Read the model definition and answer for the solid it produces. Units are mm, in the model's axes. Face numbers are marked on the shaded views. A direction names the side the tool comes from. Give positions to 0.01 mm unless a question says otherwise; leave off trailing zeros. Loops run counter-clockwise (first coordinate to the right, second up) from the corner with the lowest first, then second, coordinate; pieces in that order, holes last. Notation, with made-up numbers: (32.25, -5.75) - (85.25, -5.75) arc R22 cw to (85.25, 0.25) - close; hole circle Ø7 at (-10.5, -10). An arc over 180 degrees is marked (long way). Write item = value, one per line.
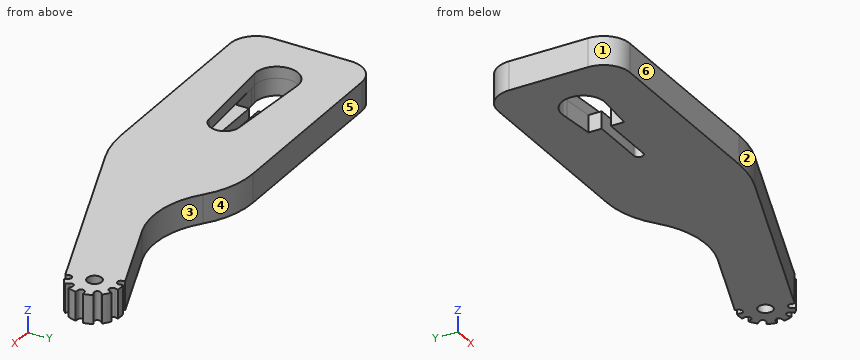
```python
from build123d import *
from build123d.topology import SkipClean

# Parameters (mm, degrees)
CROQUIS1_R              = 1.717841821
CROQUIS1_R_2            = 1.259750669
CROQUIS1_W              = 27.485469141
CROQUIS1_H              = 14.887962451
SALIENTE_EXTRUIR1_DEPTH = 5
SALIENTE_EXTRUIR2_START = -5
SALIENTE_EXTRUIR2_DEPTH = 5
CORTAR_EXTRUIR1_DEPTH   = 5
CORTAR_EXTRUIR2_DEPTH   = 2
CUT_EXTRUDE2_DEPTH      = 83.704538261
CUT_EXTRUDE5_DEPTH      = 83.704538261


with BuildPart() as part:
    # Croquis1 → Saliente-Extruir1 (new body)
    with BuildSketch(Plane(origin=(0, 0, -2.5), x_dir=(-1, 0, 0), z_dir=(0, 0, -1))):
        with BuildLine():
            Line((2.183126414, 10.199004786), (2.457799007, 10.747834714))
            ThreePointArc((2.457799007, 10.747834714), (3.150356623, 11.03498533), (3.533498829, 10.390552574))
            Line((3.533498829, 10.390552574), (3.410556906, 9.704532228))
            Line((3.410556906, 9.704532228), (36.957948904, -3.17310503))
            ThreePointArc((36.957948904, -3.17310503), (40.309989238, -4.118478177), (43.778179918, -4.437160132))
            Line((43.778179918, -4.437160132), (75.884737747, -4.437160132))
            ThreePointArc((75.884737747, -4.437160132), (79.123931349, -3.095442211), (80.46564927, 0.143751392))
            Line((80.46564927, 0.143751392), (80.46564927, 13.886485962))
            ThreePointArc((80.46564927, 13.886485962), (79.123931349, 17.125679564), (75.884737747, 18.467397485))
            Line((75.884737747, 18.467397485), (43.778179918, 18.467397485))
            ThreePointArc((43.778179918, 18.467397485), (38.923372817, 17.631925595), (34.62713443, 15.221634951))
            ThreePointArc((34.62713443, 15.221634951), (27.84817952, 12.197288027), (20.46564927, 12.971336544))
            Line((20.46564927, 12.971336544), (6.293279019, 18.411599775))
            Line((6.293279019, 18.411599775), (6.008822105, 17.843219559))
            ThreePointArc((6.008822105, 17.843219559), (5.316264489, 17.556068943), (4.933122282, 18.200501699))
            Line((4.933122282, 18.200501699), (5.041383533, 18.804603367))
            ThreePointArc((5.041383533, 18.804603367), (4.263160644, 18.876341405), (3.484068945, 18.814751339))
            Line((3.484068945, 18.814751339), (3.584448287, 18.209290101))
            ThreePointArc((3.584448287, 18.209290101), (3.192940304, 17.56990522), (2.504183677, 17.866056933))
            Line((2.504183677, 17.866056933), (2.236686818, 18.418419815))
            ThreePointArc((2.236686818, 18.418419815), (1.564924714, 18.019029169), (0.970828021, 17.511263148))
            Line((0.970828021, 17.511263148), (1.407917802, 17.080436215))
            ThreePointArc((1.407917802, 17.080436215), (1.467002194, 16.333040361), (0.735712768, 16.167791142))
            Line((0.735712768, 16.167791142), (0.194632507, 16.457431391))
            ThreePointArc((0.194632507, 16.457431391), (-0.114078519, 15.739465714), (-0.296255461, 14.9794731))
            Line((-0.296255461, 14.9794731), (0.310591317, 14.887841716))
            ThreePointArc((0.310591317, 14.887841716), (0.797699855, 14.317914702), (0.303205335, 13.754384137))
            Line((0.303205335, 13.754384137), (-0.304784058, 13.670669023))
            ThreePointArc((-0.304784058, 13.670669023), (-0.132526888, 12.9083668), (0.16680132, 12.18643894))
            Line((0.16680132, 12.18643894), (0.711610253, 12.469003179))
            ThreePointArc((0.711610253, 12.469003179), (1.440684032, 12.294237755), (1.371864517, 11.547675365))
            Line((1.371864517, 11.547675365), (0.929197275, 11.122581216))
            ThreePointArc((0.929197275, 11.122581216), (1.516626257, 10.607115987), (2.183126414, 10.199004786))
        make_face()
        with Locations(Location((46.05155145, 7.015118677, 0), (0, 0, 180))):
            Circle(CROQUIS1_R, mode=Mode.SUBTRACT)
        with Locations(Location((77.659840962, 7.015118677, 0), (0, 0, 180))):
            Circle(CROQUIS1_R, mode=Mode.SUBTRACT)
        with Locations(Location((4.233310556, 14.295527136, 0), (0, 0, 180))):
            Circle(CROQUIS1_R_2, mode=Mode.SUBTRACT)
        with Locations((61.855696206, 7.015118677)):
            Rectangle(CROQUIS1_W, CROQUIS1_H, mode=Mode.SUBTRACT)
    extrude(amount=-SALIENTE_EXTRUIR1_DEPTH)

    # Croquis2 → Saliente-Extruir2 (add)
    with BuildSketch(Plane.XY.offset(2.5).offset(SALIENTE_EXTRUIR2_START)):
        with BuildLine():
            Line((-43.778179918, -4.437160132), (-75.884737747, -4.437160132))
            ThreePointArc((-75.884737747, -4.437160132), (-79.123931349, -3.095442211), (-80.46564927, 0.143751392))
            Line((-80.46564927, 0.143751392), (-80.46564927, 13.886485962))
            ThreePointArc((-80.46564927, 13.886485962), (-79.123931349, 17.125679564), (-75.884737747, 18.467397485))
            Line((-75.884737747, 18.467397485), (-43.778179918, 18.467397485))
            Line((-43.778179918, 18.467397485), (-43.778179918, -4.437160132))
        make_face()
    extrude(amount=SALIENTE_EXTRUIR2_DEPTH)

    # Croquis3 → Cortar-Extruir1 (cut)
    with BuildSketch(Plane.XY.offset(2.5)):
        with BuildLine():
            Line((-68.86564927, 10.615118677), (-63.46564927, 10.110118677))
            Line((-63.46564927, 10.110118677), (-63.46564927, 3.920118677))
            Line((-63.46564927, 3.920118677), (-68.86564927, 3.415118677))
            ThreePointArc((-68.86564927, 3.415118677), (-72.46564927, 7.015118677), (-68.86564927, 10.615118677))
        make_face()
    extrude(amount=-CORTAR_EXTRUIR1_DEPTH, mode=Mode.SUBTRACT)

    # Croquis4 → Cortar-Extruir2 (cut)
    with BuildSketch(Plane.XY.offset(2.5)):
        with BuildLine():
            Line((-54.77859891, 9.608381518), (-69.913267682, 10.700035319))
            ThreePointArc((-69.913267682, 10.700035319), (-73.947018097, 7.015118677), (-69.913267682, 3.330202034))
            Line((-69.913267682, 3.330202034), (-54.77859891, 4.421855836))
            ThreePointArc((-54.77859891, 4.421855836), (-52.36564927, 7.015118677), (-54.77859891, 9.608381518))
        make_face()
    extrude(amount=-CORTAR_EXTRUIR2_DEPTH, mode=Mode.SUBTRACT)

    # Sketch2 → Cut-Extrude2 (cut, through all)
    with SkipClean():  # the faces are left unmerged after this step: merging them gives an invalid solid
        with BuildSketch(Plane.XY.offset(0.5)):
            with BuildLine():
                Line((-69.913267682, 10.700035319), (-68.86564927, 10.615118677))
                ThreePointArc((-68.86564927, 10.615118677), (-72.46564927, 7.015118677), (-68.86564927, 3.415118677))
                Line((-68.86564927, 3.415118677), (-69.913267682, 3.330202034))
                ThreePointArc((-69.913267682, 3.330202034), (-73.947018097, 7.015118677), (-69.913267682, 10.700035319))
            make_face()
        extrude(amount=-CUT_EXTRUDE2_DEPTH, mode=Mode.SUBTRACT)

    # Sketch5 → Cut-Extrude5 (cut, through all)
    with SkipClean():  # the faces are left unmerged after this step: merging them gives an invalid solid
        with BuildSketch(Plane.XY.offset(0.5)):
            with BuildLine():
                Line((-63.46564927, 7.815118677), (-53.96564927, 7.815118677))
                ThreePointArc((-53.96564927, 7.815118677), (-53.16564927, 7.015118677), (-53.96564927, 6.215118677))
                Line((-53.96564927, 6.215118677), (-63.46564927, 6.215118677))
                Line((-63.46564927, 6.215118677), (-63.46564927, 7.815118677))
            make_face()
        extrude(amount=-CUT_EXTRUDE5_DEPTH, mode=Mode.SUBTRACT)


solid = part.part
```
1) The mould has two halves that part along X. Classify the marked faces 1, 2, 3 and 4: pulls with the +X half, pulls with the -X half, needs draft (parallel to the pull), parting line crosses it, or undercut.
Output:
face_1 = pulls with the -X half
face_2 = pulls with the +X half
face_3 = undercut
face_4 = undercut
2) Find the intervals of material crossed by probe 1 along Y at (x, z) = (-74.5, 0.65); probe 2 along X at (y, z) = (11, 1.1); probe 3 along X at (y, z) = (10, -1.35), in increasing order.
Output:
probe_1 = -4.44 to 18.47
probe_2 = -80.47 to -3.23, -2.71 to -1.05
probe_3 = -80.47 to -72.43, -63.47 to -3.46
3) A tool of negligible diameter and unlimited length cuts with its end or side. For the marked faces 5 and 6, from which of +Z, -Z, +X, -X, +Y, -Y can it reach the whole face along a straight path? Write none if from no direction.
Output:
face_5 = +Z, -Z, -X, +Y
face_6 = +Z, -Z, +X, -X, -Y
4) A cutting plane is placed at B-B on z = -0.45. Give the number of separate pieces and of enclosed holes in the cut face, then the cut area to 3 significant figures.
Output:
separate_pieces = 1
enclosed_holes = 2
area = 1,300 mm²
5) Each of these flat-tipped pins is pushed along its axis until it touches: P1, Ø8.5, axis at x = -70.25, y = 7.02, coming from the +Z side; P2, Ø3.5, axis at x = -64.5, y = 6, coming from the +Z side; P3, Ø1.5, axis at x = -66.5, z = -2, coming from the +Y side. Where does it stop, or does it pass through?
Output:
P1 = 2.5
P2 = 0.5
P3 = 18.47
6) A cutting plane is placed at A-A on x = -62.5. Determine the outline of the cut face in (y, z).
Output:
outline = (-4.44, -2.5) - (6.22, -2.5) - (6.22, 0.5) - (3.86, 0.5) - (3.86, 2.5) - (-4.44, 2.5) - close; (7.82, -2.5) - (18.47, -2.5) - (18.47, 2.5) - (10.17, 2.5) - (10.17, 0.5) - (7.82, 0.5) - close
7) A cutting plane is placed at C-C on x = -50.5. Determine the outline of the cut face in (y, z), then the cut area to 3 significant figures.
Output:
outline = (-4.44, -2.5) - (18.47, -2.5) - (18.47, 2.5) - (-4.44, 2.5) - close
area = 115 mm²
8) A cutting plane is placed at D-D on y = -1. Determine the outline of the cut face in (x, z).
Output:
outline = (-80.32, -2.5) - (-31.3, -2.5) - (-31.3, 2.5) - (-80.32, 2.5) - close
